from build123d import *

# Parameters (mm, degrees)
SKETCH1_W               = 60
SKETCH1_H               = 60
SKETCH1_W_2             = 55
SKETCH1_H_2             = 55
BOSS_EXTRUDE1_DEPTH     = 40
SKETCH2_W               = 60
SKETCH2_H               = 60
BOSS_EXTRUDE2_DEPTH     = 2.5
BOSS_EXTRUDE3_DEPTH     = 60
CUT_EXTRUDE1_REACH      = 82.061
CUT_EXTRUDE2_DEPTH      = 81.060539593
CUT_EXTRUDE2_DEPTH_BACK = 81.060539593
SKETCH5_W               = 60
SKETCH5_H               = 41


with BuildPart() as part:
    # Sketch1 → Boss-Extrude1 (new body)
    with BuildSketch(Plane(origin=(0, 0, 0), x_dir=(1, 0, 0), z_dir=(0, 1, 0))):
        Rectangle(SKETCH1_W, SKETCH1_H)
        Rectangle(SKETCH1_W_2, SKETCH1_H_2, mode=Mode.SUBTRACT)
    extrude(amount=BOSS_EXTRUDE1_DEPTH)

    # Sketch2 → Boss-Extrude2 (add)
    with BuildSketch(Plane(origin=(0, 40, 0), x_dir=(1, 0, 0), z_dir=(0, 1, 0))):
        Rectangle(SKETCH2_W, SKETCH2_H)
    extrude(amount=BOSS_EXTRUDE2_DEPTH)

    # Sketch3 → Boss-Extrude3 (add)
    with BuildSketch(Plane(origin=(0, 0, -30), x_dir=(-1, 0, 0), z_dir=(0, 0, -1))):
        Polygon((-30, 42.5), (-28.8, 43.7), (-27.6, 42.5), (-26.4, 43.7), (-25.2, 42.5), (-24, 43.7), (-22.8, 42.5), (-21.6, 43.7), (-20.4, 42.5), (-19.2, 43.7), (-18, 42.5), (-16.8, 43.7), (-15.6, 42.5), (-14.4, 43.7), (-13.2, 42.5), (-12, 43.7), (-10.8, 42.5), (-9.6, 43.7), (-8.4, 42.5), (-7.2, 43.7), (-6, 42.5), (-4.8, 43.7), (-3.6, 42.5), (-2.4, 43.7), (-1.2, 42.5), (0, 43.7), (1.2, 42.5), (2.4, 43.7), (3.6, 42.5), (4.8, 43.7), (6, 42.5), (7.2, 43.7), (8.4, 42.5), (9.6, 43.7), (10.8, 42.5), (12, 43.7), (13.2, 42.5), (14.4, 43.7), (15.6, 42.5), (16.8, 43.7), (18, 42.5), (19.2, 43.7), (20.4, 42.5), (21.6, 43.7), (22.8, 42.5), (24, 43.7), (25.2, 42.5), (26.4, 43.7), (27.6, 42.5), (28.8, 43.7), (30, 42.5), (30, 42.170064374), (-30, 42.170064374), align=None)
    extrude(amount=-BOSS_EXTRUDE3_DEPTH)

    # Cut-Extrude1: up to this face of the body (flat: up to its plane)
    cut_extrude1_end = Plane(part.part.faces().sort_by_distance((30, 21.25, 0))[0])
    # Sketch4 → Cut-Extrude1 (cut, up to the picked face)
    with BuildSketch(Plane.ZY.offset(30), mode=Mode.PRIVATE) as cut_extrude1_sk1:
        with BuildLine():
            Line((-30, 42.5), (-30, 43.7))
            Line((-30, 43.7), (-28.8, 43.7))
            ThreePointArc((-28.8, 43.7), (-29.648528137, 43.348528137), (-30, 42.5))
        make_face()
    cut_extrude1_tool1 = split(extrude(cut_extrude1_sk1.sketch, amount=-CUT_EXTRUDE1_REACH, mode=Mode.PRIVATE), bisect_by=cut_extrude1_end, keep=Keep.BOTH, mode=Mode.PRIVATE)
    cut_extrude1 = cut_extrude1_tool1.solids().sort_by(Axis((-30, 43.431958, -29.731958), (1, 0, 0)))[0]
    add(cut_extrude1, mode=Mode.SUBTRACT)

    # Mirror1: Cut-Extrude1 across plane
    add(cut_extrude1.mirror(Plane.XY), mode=Mode.SUBTRACT)

    # Sketch5 → Cut-Extrude2 (cut, two sides: drawn at the far end of the back side and taken through both)
    with BuildSketch(Plane.XY.offset(30).offset(-CUT_EXTRUDE2_DEPTH_BACK)):
        with Locations((0, 20.5)):
            Rectangle(SKETCH5_W, SKETCH5_H)
    extrude(amount=CUT_EXTRUDE2_DEPTH + CUT_EXTRUDE2_DEPTH_BACK, mode=Mode.SUBTRACT)


solid = part.part
The listing builds one solid part. Answer for the finished solid, in the listing's coordinates (mm). Coordinates: 2 decimals unless noted, no trailing zeros.
1) A flat-ended cylindrical pin translates along its axis: pin 1 Ø8 at (x, z) = (-11.5, 12) entering from +Y. Find the tip coordinate at first contact, or state that the pin passes through.
2) Find the intervals of material crossed by L1, parallel to Z at x = -10.5, y = 42.55; L2, parallel to Y at x = -22, z = 12; L3, parallel to Y at x = 17, z = -16, in increasing order.
3) Find section A-A on y = 43.2. Give the number of separate pieces and of enclosed holes in the cut face, then the cut area to 3 significant figures.
Values:
1. pin 1: stops at y = 43.7
2. L1: z = -30 to 30
2. L2: y = 41 to 43.3
2. L3: y = 41 to 43.5
3. separate pieces: 25
3. enclosed holes: 0
3. area: 1,490 mm2
